Verification items for the finished model (mm, model axes). A direction names the side the tool comes from. Round coordinates to 2 decimals unless told otherwise and drop trailing zeros. Write each loop counter-clockwise with the first axis right and the second up, starting at its lowest first coordinate (ties: lowest second). Pieces come first, ordered by that corner, then holes. Notation, with made-up numbers: (85.5, 3) -> (95.5, 3) arc R28 ccw to (95.5, 40) -> close; hole circle Ø6 at (76.5, 28.5). An arc over 180 degrees is marked (long way). Use CSV: the item, a comma, the result in double quotes.
```python
from build123d import *

# Parameters (mm, degrees)
SKETCH_1_R      = 12.2
EXTRUDE_1_DEPTH = 21
FILLET_1_R      = 1
SKETCH_2_R      = 3.5
EXTRUDE_2_DEPTH = 2.5
SKETCH_3_R      = 2
EXTRUDE_3_DEPTH = 9


with BuildPart() as part:
    # 草图1 → 凸台-拉伸1 (new body)
    with BuildSketch(Plane(origin=(0, 0, 0), x_dir=(0, 0, -1), z_dir=(1, 0, 0))):
        with Locations(Location((0, 0, 0), (0, 0, 180))):
            Circle(SKETCH_1_R)
    extrude(amount=EXTRUDE_1_DEPTH)

    # 圆角1
    fillet_1_edges = [part.edges().sort_by_distance(p)[0] for p in [
        (0, 0, -12.2),
        (21, 0, -12.2),
    ]]
    fillet(fillet_1_edges, radius=FILLET_1_R)

    # 草图2 → 凸台-拉伸2 (add)
    with BuildSketch(Plane.ZY):
        with Locations(Location((0, 0, 0), (0, 0, 180))):
            Circle(SKETCH_2_R)
    extrude(amount=EXTRUDE_2_DEPTH)

    # 草图3 → 凸台-拉伸3 (add)
    with BuildSketch(Plane.ZY.offset(2.5)):
        Circle(SKETCH_3_R)
    extrude(amount=EXTRUDE_3_DEPTH)


solid = part.part
```
Q1. Section check C-C (x = 4). Record the cut outline in (y, z).
Filled in:
outline,"circle Ø24.4 at (0, 0)"
Q2. Mould release check, pull along Y, two halves, no side actions. Record for faces 1 (the cylindrical face through (10.37, -0.54, -12.19)), 2 (the flat face through (0, -3, -3)): released by +Y, released by -Y, zero draft, split by the parting line, or undercut.
Filled in:
face 1,"split by the parting line"
face 2,"zero draft"
Q3. Access from +Z, -Z, +X, -X, +Y, -Y to the whole of each face (thin tool, end or side, straight path). Record for faces 3 (the flat face through (21, 0, 0)), 4 (the cylindrical face through (-1.232, 1.341, -3.233)).
Filled in:
face 3,"+Z, -Z, +X, +Y, -Y"
face 4,"-X"
Q4. Section check A-A (z = 0). Record the cut outline in (x, y).
Filled in:
outline,"(-11.5, -2) -> (-2.5, -2) -> (-2.5, -3.5) -> (0, -3.5) -> (0, -11.2) arc R1 ccw to (1, -12.2) -> (20, -12.2) arc R1 ccw to (21, -11.2) -> (21, 11.2) arc R1 ccw to (20, 12.2) -> (1, 12.2) arc R1 ccw to (0, 11.2) -> (0, 3.5) -> (-2.5, 3.5) -> (-2.5, 2) -> (-11.5, 2) -> close"
Q5. Go/stop test with flat-tipped pins: P1, Ø1, axis at x = 11.5, z = 2, coming from the -Y side; P2, Ø6, axis at y = 1, z = -9, coming from the -X side; P3, Ø5, axis at x = -1, y = 4, coming from the -Z side. Record where each tip stops, or that it passes through.
Filled in:
P1,"y = -12.11"
P2,"x = 0"
P3,"z = -11.97"
Q6. Material ranges on L1, parallel to X at y = -8.25, z = 2.5; L2, parallel to Z at x = 19, y = -0.25; L3, parallel to Z at x = 2.5, y = 10.5, recorded low to high.
Filled in:
L1,"0 to 21"
L2,"-12.2 to 12.2"
L3,"-6.21 to 6.21"
